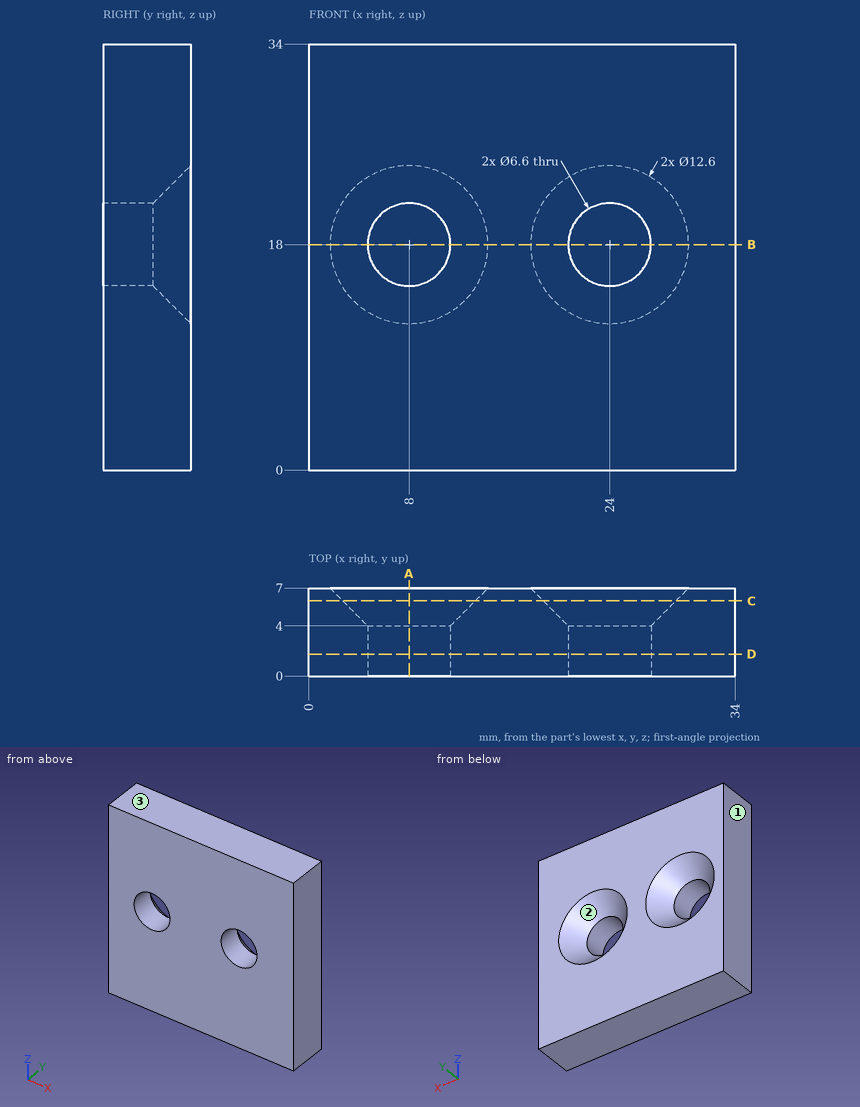
The figure shows three views and two pictorial views of one solid part (mm, origin at its lowest corner). Answer the questions. Round coordinates to 2 decimals unless told otherwise and drop trailing zeros. Write each loop counter-clockwise with the first axis right and the second up, starting at its lowest first coordinate (ties: lowest second). Pieces come first, ordered by that corner, then holes. Notation, with made-up numbers: (36, 23.5) - (51, 23.5) arc R13 cw to (51, 32.5) - close; hole circle Ø8 at (51.5, 88.25). An arc over 180 degrees is marked (long way). One line per question, with ' | ' between items. Start each with the question number.
1. Section C-C (y = 6) is taken. Determine the outline of the cut face in (x, z), and give its area (3 significant figures).
2. Section A-A (x = 8) is taken. Determine the outline of the cut face in (y, z).
3. Each of these flat-tipped pins is pushed along its axis until it touches: pin 1 (6 mm diameter, centred on x = 8, z = 18, fed in from -Y); pin 2 (4 mm diameter, centred on y = 4, z = 8.5, fed in from -X). Where does it stop, or does it pass through?
4. For a pull along X with two mould halves and no side action, classify the marked faces 1, 2 and 3 as +X half, -X half, draft (parallel to the pull), parting line (faces both ways), or undercut.
5. Section B-B (z = 18) is taken. Determine the outline of the cut face in (x, y).
6. Find the intervals of material crossed by probe 1 along X at (y, z) = (0.8, 18); probe 2 along Z at (x, y) = (24, 1.15); probe 3 along X at (y, z) = (2.5, 19.5), in increasing order. Write a range as [from, to].
7. Section D-D (y = 1.75) is taken. Determine the outline of the cut face in (x, z), and give its area (3 significant figures).
Filled in:
1) outline: (0, 0) - (34, 0) - (34, 34) - (0, 34) - close; hole circle Ø10.6 at (8, 18); hole circle Ø10.6 at (24, 18) | area: 980 mm²
2) outline: (0, 0) - (7, 0) - (7, 11.7) - (4, 14.7) - (0, 14.7) - close; (0, 21.3) - (4, 21.3) - (7, 24.3) - (7, 34) - (0, 34) - close
3) pin 1: through | pin 2: x = 0
4) face 1: -X half | face 2: undercut | face 3: draft
5) outline: (0, 0) - (4.7, 0) - (4.7, 4) - (1.7, 7) - (0, 7) - close; (11.3, 0) - (20.7, 0) - (20.7, 4) - (17.7, 7) - (14.3, 7) - (11.3, 4) - close; (27.3, 0) - (34, 0) - (34, 7) - (30.3, 7) - (27.3, 4) - close
6) probe 1: [0, 4.7], [11.3, 20.7], [27.3, 34] | probe 2: [0, 14.7], [21.3, 34] | probe 3: [0, 5.06], [10.94, 21.06], [26.94, 34]
7) outline: (0, 0) - (34, 0) - (34, 34) - (0, 34) - close; hole circle Ø6.6 at (8, 18); hole circle Ø6.6 at (24, 18) | area: 1,090 mm²
